Could you check a few things on this model? Use its own coordinates, in mm. A direction names the side the tool comes from. Round coordinates to 2 decimals unless told otherwise and drop trailing zeros. Write each loop counter-clockwise with the first axis right and the second up, starting at its lowest first coordinate (ties: lowest second). Pieces come first, ordered by that corner, then holes. Notation, with made-up numbers: (37, -28) -> (57, -28) arc R20 cw to (57, -24) -> close; hole circle Ø10 at (50, 86.25). An arc over 180 degrees is marked (long way). Answer in a Markdown table with one row per item. Add a question column.
```python
from build123d import *

# Parameters (mm, degrees)
SKETCH1_W            = 90
SKETCH1_H            = 70
BOSS_EXTRUDE1_DEPTH  = 25
SHELL1_T             = -2.5
SKETCH2_W            = 25
SKETCH2_H            = 70
CUT_EXTRUDE1_DEPTH   = 16
SKETCH3_W            = 20
SKETCH3_H            = 2.5
BOSS_EXTRUDE2_DEPTH  = 25
SKETCH4_W            = 20
SKETCH4_H            = 2.5
BOSS_EXTRUDE3_DEPTH  = 10
FILLET1_R            = 8
FILLET1_OF_MIRROR2_R = 8
FILLET3_R            = 10
FILLET4_R            = 5
FILLET5_R            = 0.5


with BuildPart() as part:
    # Sketch1 → Boss-Extrude1 (new body)
    with BuildSketch(Plane.XY):
        Rectangle(SKETCH1_W, SKETCH1_H)
    extrude(amount=BOSS_EXTRUDE1_DEPTH)

    # Shell1
    shell1_openings = [part.faces().sort_by_distance(p)[0] for p in [
        (0, 35, 12.5),
    ]]
    offset(amount=SHELL1_T, openings=shell1_openings, kind=Kind.INTERSECTION)

    # Sketch2 → Cut-Extrude1 (cut)
    with BuildSketch(Plane.XY.offset(25)):
        Rectangle(SKETCH2_W, SKETCH2_H)
    extrude(amount=-CUT_EXTRUDE1_DEPTH, mode=Mode.SUBTRACT)

    # Sketch3 → Boss-Extrude2 (add)
    with BuildSketch(Plane.XY.offset(25)):
        with Locations((-28.75, -33.75)):
            Rectangle(SKETCH3_W, SKETCH3_H)
    boss_extrude2 = extrude(amount=BOSS_EXTRUDE2_DEPTH)

    # Sketch4 → Boss-Extrude3 (add)
    with BuildSketch(Plane(origin=(0, -32.5, 0), x_dir=(1, 0, 0), z_dir=(0, 1, 0))):
        with Locations((-28.75, -48.75)):
            Rectangle(SKETCH4_W, SKETCH4_H)
    boss_extrude3 = extrude(amount=BOSS_EXTRUDE3_DEPTH)

    # Fillet1
    fillet1_edges = [part.edges().sort_by_distance(p)[0] for p in [
        (-18.75, -22.5, 48.75),
        (-38.75, -22.5, 48.75),
    ]]
    fillet(fillet1_edges, radius=FILLET1_R)

    # Mirror2: Boss-Extrude2, Boss-Extrude3 across plane
    add(boss_extrude2.mirror(Plane(origin=(0, 0, 0), x_dir=(0, 0, 1), z_dir=(1, 0, 0))))
    add(boss_extrude3.mirror(Plane(origin=(0, 0, 0), x_dir=(0, 0, 1), z_dir=(1, 0, 0))))

    # Fillet1 of Mirror2
    fillet1_of_mirror2_edges = [part.edges().sort_by_distance(p)[0] for p in [
        (18.75, -22.5, 48.75),
        (38.75, -22.5, 48.75),
    ]]
    fillet(fillet1_of_mirror2_edges, radius=FILLET1_OF_MIRROR2_R)

    # Fillet3
    fillet3_edges = [part.edges().sort_by_distance(p)[0] for p in [
        (-12.5, 35, 23.75),
        (12.5, 35, 23.75),
    ]]
    fillet(fillet3_edges, radius=FILLET3_R)

    # Fillet4
    fillet4_edges = [part.edges().sort_by_distance(p)[0] for p in [
        (-12.5, -33.75, 9),
        (12.5, -33.75, 9),
    ]]
    fillet(fillet4_edges, radius=FILLET4_R)

    # Fillet5
    fillet5_edges = [part.edges().sort_by_distance(p)[0] for p in [
        (-12.5, -3.75, 22.5),
        (-12.5, -5, 25),
        (-33.75, 35, 25),
        (-15.428932188, 32.071067812, 25),
        (-32.5, 35, 22.5),
        (-15.428932188, 32.071067812, 22.5),
        (15.428932188, 32.071067812, 25),
        (-45, 0, 25),
        (15.428932188, 32.071067812, 22.5),
        (0, -32.5, 9),
        (-12.5, -32.5, 18.25),
        (11.035533906, -32.5, 10.464466094),
        (-11.035533906, -32.5, 10.464466094),
        (42.5, 1.25, 2.5),
        (42.5, -32.5, 12.5),
        (0, 35, 2.5),
        (42.5, 35, 12.5),
        (-42.5, 1.25, 2.5),
        (-42.5, 35, 12.5),
        (0, -32.5, 2.5),
        (-42.5, -32.5, 12.5),
        (32.5, 35, 22.5),
        (-42.5, 1.25, 22.5),
        (-27.5, -32.5, 22.5),
        (27.5, -32.5, 22.5),
        (12.5, -3.75, 22.5),
        (12.5, -32.5, 18.25),
        (12.5, -5, 25),
        (45, 0, 25),
        (0, -35, 0),
        (-45, 0, 0),
        (0, 35, 0),
        (45, 0, 0),
        (45, -35, 12.5),
        (-45, -35, 12.5),
        (-45, 35, 12.5),
        (45, 35, 12.5),
        (33.75, 35, 25),
    ]]
    fillet(fillet5_edges, radius=FILLET5_R)


solid = part.part
```
(1) Suppose I cut it at A-A, the plane z = 15. Please give me the cut outline in (x, y), then the cut area to 3 significant figures.
(2) For P1, Ø10, axis at x = -21.5, y = -20, coming from the +Z side; P2, Ø12, axis at y = -24, z = 31.5, coming from the -X side; P3, Ø3, axis at x = 29, z = 48.5, coming from the +Y side; P4, Ø10, axis at x = -28.5, z = 39.5, coming from the +Y side, each with a flat end and sliding along its axis, tell me the tip position at first contact or that it passes through.
(3) Suppose I cut it at B-B, the plane x = -1.5. Please give me the cut outline in (y, z).
(4) I need wall thicknesses on L1, parallel to Z at x = -32.5, y = -29.5; L2, parallel to Z at x = -14, y = -11; L3, parallel to X at y = 18, z = 12. Which ranges of each line are inside material? Lowest first, please.
(5) On a 3-axis mill with a long thin cutter (end or side, diameter ignored), from which of +Z, -Z, +X, -X, +Y, -Y can I reach the whole of each face in a straight line? I mean faces 4 (the face through (-29, -28, 47.5)), 5 (the face through (-29, -22.5, 49)), 6 (the face through (15.35, 31.99, 23.74)), 7 (the face through (-28, 2, 22.5)), 8 (the face through (-12.5, -9.6, 23.2)). Say none if no direction works.
(6) Suppose I cut it at D-D, the plane z = 5. Please give me the cut outline in (x, y).
(7) If we mould it in two halves opening along X, with no side actions, what happens to faces 1 (the face through (-38.75, -34, 38)), 2 (the face through (-1, 2, 2.5)), 3 (the face through (29, -32.5, 36))? For each: pulls with the +X half, pulls with the -X half, needs draft (parallel to the pull), parting line crosses it, or undercut.
(8) Suppose I cut it at C-C, the plane y = 16. Please give me the cut outline in (x, z).
Response:
| question | item | result |
|---|---|---|
| 1 | outline | (-45, -34.5) arc R0.5 ccw to (-44.5, -35) -> (-12.5, -35) -> (-12.5, -33) arc R0.5 ccw to (-13, -32.5) -> (-42, -32.5) arc R0.5 cw to (-42.5, -32) -> (-42.5, 34.5) arc R0.5 ccw to (-43, 35) -> (-44.5, 35) arc R0.5 ccw to (-45, 34.5) -> close; (12.5, -35) -> (44.5, -35) arc R0.5 ccw to (45, -34.5) -> (45, 34.5) arc R0.5 ccw to (44.5, 35) -> (43, 35) arc R0.5 ccw to (42.5, 34.5) -> (42.5, -32) arc R0.5 cw to (42, -32.5) -> (13, -32.5) arc R0.5 ccw to (12.5, -33) -> close |
| 1 | area | 500 mm² |
| 2 | P1 | z = 50 |
| 2 | P2 | through |
| 2 | P3 | y = -22.5 |
| 2 | P4 | y = -32.5 |
| 3 | outline | (-35, 0.5) arc R0.5 ccw to (-34.5, 0) -> (34.5, 0) arc R0.5 ccw to (35, 0.5) -> (35, 2) arc R0.5 ccw to (34.5, 2.5) -> (-32, 2.5) arc R0.5 cw to (-32.5, 3) -> (-32.5, 8.5) arc R0.5 ccw to (-33, 9) -> (-35, 9) -> close |
| 4 | L1 | 0 to 2.5, 22.5 to 25, 47.5 to 50 |
| 4 | L2 | 0 to 2.5, 22.5 to 25 |
| 4 | L3 | -45 to -42.5, 42.5 to 45 |
| 5 | face 4 | +X, -X, +Y |
| 5 | face 5 | +Z, +X, -X, +Y |
| 5 | face 6 | +Z, +Y |
| 5 | face 7 | +Y |
| 5 | face 8 | +Z, +Y, -Y |
| 6 | outline | (-45, -34.5) arc R0.5 ccw to (-44.5, -35) -> (44.5, -35) arc R0.5 ccw to (45, -34.5) -> (45, 34.5) arc R0.5 ccw to (44.5, 35) -> (43, 35) arc R0.5 ccw to (42.5, 34.5) -> (42.5, -32) arc R0.5 cw to (42, -32.5) -> (-42, -32.5) arc R0.5 cw to (-42.5, -32) -> (-42.5, 34.5) arc R0.5 ccw to (-43, 35) -> (-44.5, 35) arc R0.5 ccw to (-45, 34.5) -> close |
| 7 | face 1 | pulls with the -X half |
| 7 | face 2 | undercut |
| 7 | face 3 | needs draft |
| 8 | outline | (-45, 0.5) arc R0.5 ccw to (-44.5, 0) -> (44.5, 0) arc R0.5 ccw to (45, 0.5) -> (45, 24.5) arc R0.5 ccw to (44.5, 25) -> (13, 25) arc R0.5 ccw to (12.5, 24.5) -> (12.5, 23) arc R0.5 ccw to (13, 22.5) -> (42.5, 22.5) -> (42.5, 3) arc R0.5 cw to (42, 2.5) -> (-42, 2.5) arc R0.5 cw to (-42.5, 3) -> (-42.5, 22) arc R0.5 cw to (-42, 22.5) -> (-13, 22.5) arc R0.5 ccw to (-12.5, 23) -> (-12.5, 24.5) arc R0.5 ccw to (-13, 25) -> (-44.5, 25) arc R0.5 ccw to (-45, 24.5) -> close |
